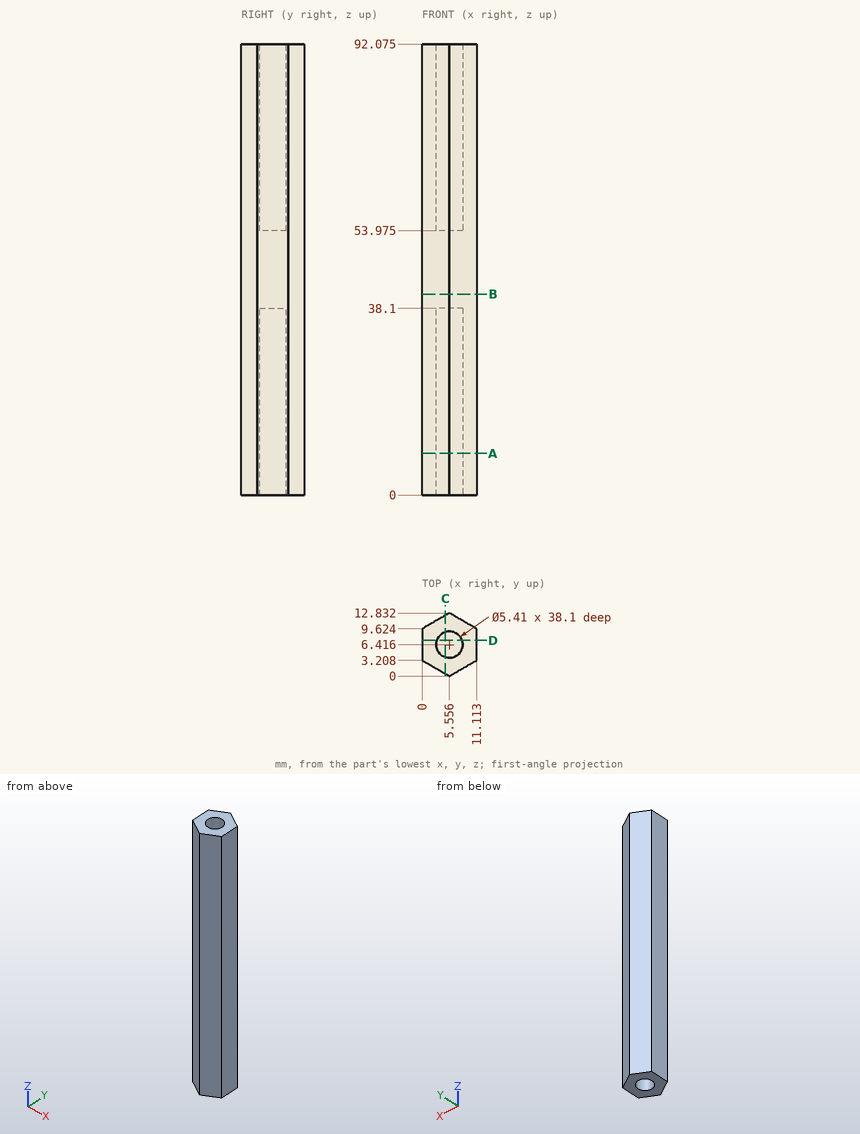
Input: dimensioned drawing with shaded views. Units: mm. Origin: part minimum x, y, z. Coordinates: 2 decimals unless noted, no trailing zeros. Loops run counter-clockwise (first coordinate to the right, second up) from the corner with the lowest first, then second, coordinate; pieces in that order, holes last. Notation, with made-up numbers: M 64.5,66.5 L 81.5,66.5 A20 ccw 81.5,79.5 Z; hole C -34,-1 d1. An arc over 180 degrees is marked long. Use a Markdown table: item, result. Add a question column.
1) Pin query (flat end, axial travel): P1, Ø4.5, axis at x = 5.56, y = 6.42, coming from the -Z side; P2, Ø5, axis at x = 5.56, y = 6.42, coming from the +Z side (1 decimal); P3, Ø2, axis at x = 3, z = 45, coming from the -Y side. Return the tip coordinate at first contact, or that it passes through.
2) Section D-D, the plane y = 7.25. Return the cut outline in (x, z) (1 decimal).
3) Section C-C, the plane x = 4.75. Return the cut outline in (y, z) (1 decimal).
4) Section B-B, the plane z = 41. Return the cut outline in (x, y), plus the area to 3 significant figures.
5) Section A-A, the plane z = 8.5. Return the cut outline in (x, y) (1 decimal).
6) Line query: L1, parallel to Y at x = 5.25, z = 8.5 (1 decimal); L2, parallel to X at y = 7.5, z = 74 (1 decimal); L3, parallel to Z at x = 5, y = 8 (1 decimal). Output: solid intervals per line, ascending. Write a range as from..to.
Answer below:
| question | item | result |
|---|---|---|
| 1 | P1 | z = 38.1 |
| 1 | P2 | z = 54 |
| 1 | P3 | y = 0.9 |
| 2 | outline | M 0,0 L 3,0 L 3,38.1 L 8.1,38.1 L 8.1,0 L 11.1,0 L 11.1,92.1 L 8.1,92.1 L 8.1,54 L 3,54 L 3,92.1 L 0,92.1 Z |
| 3 | outline | M 0.5,0 L 3.8,0 L 3.8,38.1 L 9,38.1 L 9,0 L 12.4,0 L 12.4,92.1 L 9,92.1 L 9,54 L 3.8,54 L 3.8,92.1 L 0.5,92.1 Z |
| 4 | outline | M 0,3.21 L 5.56,0 L 11.11,3.21 L 11.11,9.62 L 5.56,12.83 L 0,9.62 Z |
| 4 | area | 107 mm2 |
| 5 | outline | M 0,3.2 L 5.6,0 L 11.1,3.2 L 11.1,9.6 L 5.6,12.8 L 0,9.6 Z; hole C 5.6,6.4 d5.4 |
| 6 | L1 | 0.2..3.7, 9.1..12.7 |
| 6 | L2 | 0..3.1, 8..11.1 |
| 6 | L3 | 38.1..54 |
